Geometry check sheet. Reference: drawing and pictorial views, mm from the part's lowest x, y, z. A direction names the side the tool comes from. Round coordinates to 2 decimals unless told otherwise and drop trailing zeros. Order: outer loops, then holes, each group sorted by start corner. A loop starts at its lowest first (then second) coordinate and runs counter-clockwise, first axis right, second up.
(1) Release check for a two-part mould opening along Z. For the marked faces 1, 2, 3 and 4 record: +Z half, -Z half, draft (parallel to the pull), parting line (faces both ways), or undercut.
(2) Sectioned sample at C-C (z = 7.5). Record the boundary of the cut face in (x, y).
(3) Sectioned sample at B-B (x = 27.5). Record the boundary of the cut face in (y, z).
(4) Sectioned sample at D-D (y = 6). Record the boundary of the cut face in (x, z).
(5) Go/stop test with flat-tipped pins: pin 1 (2 mm diameter, centred on y = 5, z = 10, fed in from -X); pin 2 (0.9 mm diameter, centred on x = 28, z = 8, fed in from -Y). Record where each tip stops, or that it passes through.
(6) Sectioned sample at A-A (y = 4). Record the boundary of the cut face in (x, z), plus the area to 3 significant figures.
(7) Set-up check for the marked faces 5, 6 and 7: record each of +Z, -Z, +X, -X, +Y, -Y from which the full face is reachable in a straight line by a thin tool's end or side.
(8) Material ranges on line 1 along X through (y, z) = (2, 3.75); line 2 along Z through (x, y) = (2.5, 2.9); line 3 along Y through (x, z) = (10.25, 11.5), recorded low to high.
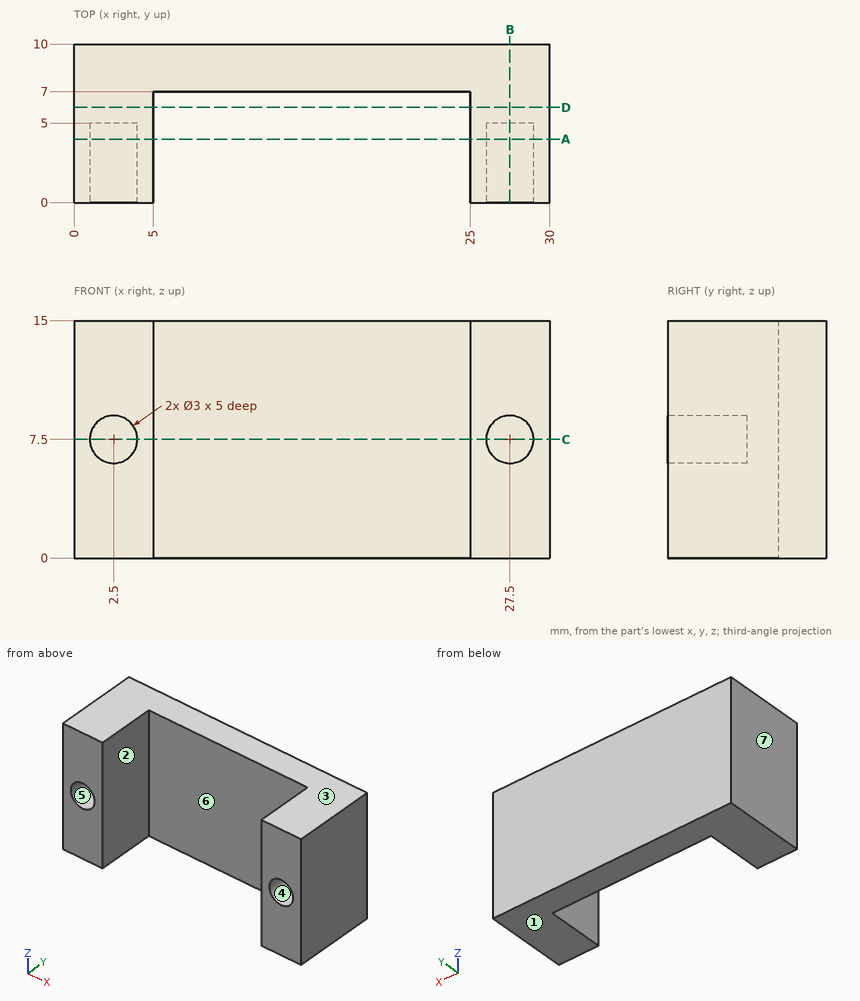
Answer below:
1. face 1: -Z half
1. face 2: draft
1. face 3: +Z half
1. face 4: undercut
2. outline: (0, 0) - (1, 0) - (1, 5) - (4, 5) - (4, 0) - (5, 0) - (5, 7) - (25, 7) - (25, 0) - (26, 0) - (26, 5) - (29, 5) - (29, 0) - (30, 0) - (30, 10) - (0, 10) - close
3. outline: (0, 0) - (10, 0) - (10, 15) - (0, 15) - (0, 9) - (5, 9) - (5, 6) - (0, 6) - close
4. outline: (0, 0) - (5, 0) - (5, 15) - (0, 15) - close; (25, 0) - (30, 0) - (30, 15) - (25, 15) - close
5. pin 1: stops at x = 0
5. pin 2: stops at y = 5
6. outline: (0, 0) - (5, 0) - (5, 15) - (0, 15) - close; (25, 0) - (30, 0) - (30, 15) - (25, 15) - close; hole circle Ø3 at (2.5, 7.5); hole circle Ø3 at (27.5, 7.5)
6. area: 136 mm2
7. face 5: -Y
7. face 6: +Z, -Z, -Y
7. face 7: +Z, -Z, -X, +Y, -Y
8. line 1: x = 0 to 5, 25 to 30
8. line 2: z = 0 to 6, 9 to 15
8. line 3: y = 7 to 10
